Verification items for the finished model (mm, model axes). Face numbers are marked on the shaded views. A direction names the side the tool comes from. Coordinates: 2 decimals unless noted, no trailing zeros. Order: outer loops, then holes, each group sorted by start corner. A loop starts at its lowest first (then second) coordinate and runs counter-clockwise, first axis right, second up. Notation, with made-up numbers: (9.25, 12) -> (64.25, 12) arc R13 cw to (64.25, 27) -> close; hole circle Ø10 at (55.5, 56.5). An arc over 180 degrees is marked (long way). Write each question's results on one line, items separated by ' | '. Start each with the question number.
(1) Set-up check for the marked faces 4, 5 and 6: record each of +Z, -Z, +X, -X, +Y, -Y from which the full face is reachable in a straight line by a thin tool's end or side.
(2) Cross-section at D-D on z = 7.61. Enter the section's corners in (x, y) (3 decimals).
(3) Cross-section at C-C on x = -11. Enter the section's corners in (y, z), and give its area (3 significant figures).
(4) Cross-section at A-A on x = -17.5. Enter the section's corners in (y, z), and give its area (3 significant figures).
(5) Draft check along Z on the marked faces 1, 2 and 3. Enter one of: +Z half, -Z half, draft (parallel to the pull), parting line (faces both ways), or undercut.
(6) Go/stop test with flat-tipped pins: pin 1 (3 mm diameter, centred on y = -3.5, z = 8.5, fed in from +X); pin 2 (2 mm diameter, centred on y = 1, z = 6.5, fed in from -X); pin 3 (1.5 mm diameter, centred on y = 2, z = 5.5, fed in from +X). Record where each tip stops, or that it passes through.
(7) Thickness scan on probe 1 along Y at (x, z) = (-17.5, 13.5); probe 2 along Y at (x, z) = (17.5, 0.25); probe 3 along X at (y, z) = (-0.25, 1.75). Record the ranges inside material, lowest first. Write a range as [from, to].
(8) Cross-section at B-B on y = 0. Give the number of separate pieces and of enclosed holes in the cut face, and give its area (3 significant figures).
```python
from build123d import *

# Parameters (mm, degrees)
PAD_DEPTH            = 5
SKETCH001_R          = 4
POCKET_DEPTH         = 5
SKETCH002_R          = 3
POCKET001_DEPTH      = 5
CHAMFER_SIZE         = 1.5
POCKET002_DEPTH      = 30.111
POCKET002_DEPTH_BACK = -30.111


with BuildPart() as part:
    # Sketch → Pad (new body, symmetric)
    with BuildSketch(Plane.XZ):
        with BuildLine():
            Line((-29.11, 14.64), (29.11, 14.64))
            ThreePointArc((29.11, 12.64), (30.11, 13.64), (29.11, 14.64))
            Line((29.11, 12.64), (8.045, 12.64))
            ThreePointArc((8.045, 12.64), (3.015, 7.61), (8.045, 2.58))
            Line((8.045, 2.58), (23.65, 2.58))
            Line((23.65, 2.58), (23.65, 0))
            Line((23.65, 0), (-23.65, 0))
            Line((-23.65, 0), (-23.65, 2.58))
            Line((-23.65, 2.58), (-8.045, 2.58))
            ThreePointArc((-8.045, 2.58), (-3.015, 7.61), (-8.045, 12.64))
            Line((-8.045, 12.64), (-29.11, 12.64))
            ThreePointArc((-29.11, 14.64), (-30.11, 13.64), (-29.11, 12.64))
        make_face()
    extrude(amount=PAD_DEPTH, both=True)

    # Sketch001 → Pocket (cut)
    with BuildSketch(Plane.XY.offset(15)):
        with Locations((-17.5, 0)):
            Circle(SKETCH001_R)
        with Locations((17.5, 0)):
            Circle(SKETCH001_R)
    extrude(amount=-POCKET_DEPTH, mode=Mode.SUBTRACT)

    # Sketch002 → Pocket001 (cut)
    with BuildSketch(Plane.XY.offset(3)):
        with Locations((-17.5, 0)):
            Circle(SKETCH002_R)
        with Locations((17.5, 0)):
            Circle(SKETCH002_R)
    extrude(amount=-POCKET001_DEPTH, mode=Mode.SUBTRACT)

    # Chamfer
    chamfer_edges = [part.edges().sort_by_distance(p)[0] for p in [
        (-20.5, 0, 2.58),
        (14.5, 0, 2.58),
    ]]
    chamfer(chamfer_edges, length=CHAMFER_SIZE)

    # Sketch003 → Pocket002 (cut, two sides)
    with BuildSketch(Plane.YZ) as pocket002_sk:
        with BuildLine():
            ThreePointArc((-7.064252, 16.860308), (0, 13.328536), (7.064252, 16.860308))
            Line((-7.064252, 16.860308), (7.064252, 16.860308))
        make_face()
    extrude(amount=-POCKET002_DEPTH, mode=Mode.SUBTRACT)
    extrude(pocket002_sk.sketch, amount=-POCKET002_DEPTH_BACK, mode=Mode.SUBTRACT)


solid = part.part
```
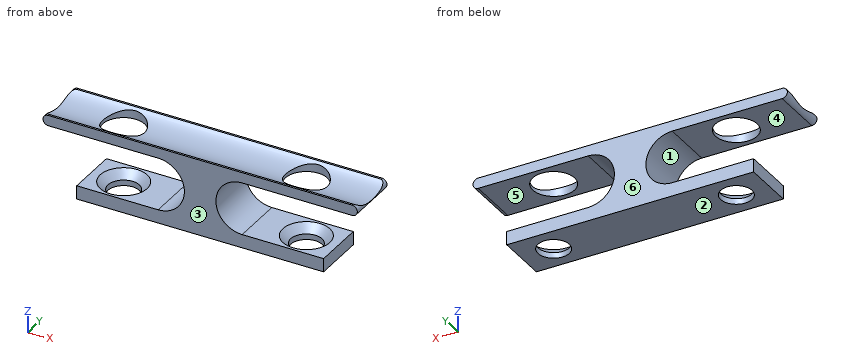
Results are:
1) face 4: -X, +Y, -Y | face 5: +X, +Y, -Y | face 6: +Z, -Z, +X, -X, +Y
2) outline: (-3.015, -5) -> (3.015, -5) -> (3.015, 5) -> (-3.015, 5) -> close
3) outline: (-5, 0) -> (5, 0) -> (5, 2.58) -> (-5, 2.58) -> close; (-5, 12.64) -> (5, 12.64) -> (5, 14.64) -> (4.63, 14.64) arc R8.83 cw to (-4.63, 14.64) -> (-5, 14.64) -> close | area: 37.6 mm2
4) outline: (-5, 0) -> (-3, 0) -> (-3, 1.08) -> (-4.5, 2.58) -> (-5, 2.58) -> close; (-5, 12.64) -> (-4, 12.64) -> (-4, 14.29) arc R8.83 cw to (-4.63, 14.64) -> (-5, 14.64) -> close; (3, 0) -> (5, 0) -> (5, 2.58) -> (4.5, 2.58) -> (3, 1.08) -> close; (4, 12.64) -> (5, 12.64) -> (5, 14.64) -> (4.63, 14.64) arc R8.83 cw to (4, 14.29) -> close | area: 11.8 mm2
5) face 1: undercut | face 2: -Z half | face 3: draft
6) pin 1: stops at x = 3.62 | pin 2: stops at x = -3.48 | pin 3: stops at x = 3.91
7) probe 1: y = [-5, -4], [4, 5] | probe 2: y = [-5, -3], [3, 5] | probe 3: x = [-23.65, -21.16], [-13.84, 13.84], [21.16, 23.65]
8) separate pieces: 5 | enclosed holes: 0 | area: 199 mm2
